Read the model definition and answer for the solid it produces. Units are mm, in the model's axes. Give positions to 0.01 mm unless a question says otherwise; leave off trailing zeros. Write each loop counter-clockwise with the first axis right and the second up, starting at its lowest first coordinate (ties: lowest second). Pieces come first, ordered by that corner, then holes. Notation, with made-up numbers: (75, 7.25) -> (121, 7.25) arc R27 cw to (121, 31.25) -> close; hole circle Ø9 at (75.5, 21.25). An arc over 180 degrees is marked (long way). Write item = value, one per line.
from build123d import *

# Parameters (mm, degrees)
F0_R     = 117.5
F0_R_2   = 11
F0_R_3   = 21.5
F1_DEPTH = 5
F2_R     = 7
F3_DEPTH = 5.001
F4_R     = 4
F5_DEPTH = 5.001


with BuildPart() as f1:
    # F0 (on Top) → F1 (new body)
    with BuildSketch(Plane.XY):
        Circle(F0_R)
        with Locations((7, -36)):
            Circle(F0_R_2, mode=Mode.SUBTRACT)
        with Locations((-17, 0)):
            Circle(F0_R_3, mode=Mode.SUBTRACT)
        with Locations((7, 36)):
            Circle(F0_R_2, mode=Mode.SUBTRACT)
    extrude(amount=F1_DEPTH)

    # F2 (on face) → F3 (cut, through all)
    with BuildSketch(Plane(origin=(0, 0, 0), x_dir=(1, 0, 0), z_dir=(0, 0, -1))):
        with Locations((-100, 0)):
            Circle(F2_R)
        with Locations((0, 100)):
            Circle(F2_R)
        with Locations((100, 0)):
            Circle(F2_R)
        with Locations((0, -100)):
            Circle(F2_R)
    extrude(amount=-F3_DEPTH, mode=Mode.SUBTRACT)

    # F4 (on face) → F5 (cut, through all)
    with BuildSketch(Plane.XY.offset(5)):
        with Locations((38, 0)):
            Circle(F4_R)
    extrude(amount=-F5_DEPTH, mode=Mode.SUBTRACT)


solid = f1.part
(1) The part is cut by section D-D on x = -43.5. Determine the outline of the cut face in (y, z).
Checks:
outline = (-109.15, 0) -> (109.15, 0) -> (109.15, 5) -> (-109.15, 5) -> close
(2) The part is cut by section A-A on x = -17. Determine the outline of the cut face in (y, z), plus the area to 3 significant figures.
Checks:
outline = (-116.26, 0) -> (-21.5, 0) -> (-21.5, 5) -> (-116.26, 5) -> close; (21.5, 0) -> (116.26, 0) -> (116.26, 5) -> (21.5, 5) -> close
area = 948 mm²
(3) For a pull along Y with two mould halves and no side action, classify faces 1 (the cylindrical face through (-0.91, 93.06, 2.46)), 2 (the flat face through (24, 2, 0)), 3 (the cylindrical face through (-15.3, 116.5, 2.5)) as released by +Y, released by -Y, zero draft, split by the parting line, or undercut.
Checks:
face_1 = undercut
face_2 = zero draft
face_3 = split by the parting line
(4) Consider L1, parallel to X at y = 6, z = 1.1; L2, parallel to Y at x = 9, z = 2.5; L3, parallel to X at y = -1.5, z = 3.5. Determine where each line is inside the solid, lowest interval first.
Checks:
L1 = -117.35 to -103.61, -96.39 to -37.65, 3.65 to 96.39, 103.61 to 117.35
L2 = -117.15 to -46.82, -25.18 to 25.18, 46.82 to 117.15
L3 = -117.49 to -106.84, -93.16 to -38.45, 4.45 to 34.29, 41.71 to 93.16, 106.84 to 117.49
(5) Given P1, Ø3, axis at y = 30.5, z = 4, coming from the -X side, flat-ended and moving along its own axis, determine where the tip first touches the part or whether it passes through.
Checks:
P1 = -113.87
(6) The part is cut by section B-B on y = -100. Determine the outline of the cut face in (x, z).
Checks:
outline = (-61.69, 0) -> (-7, 0) -> (-7, 5) -> (-61.69, 5) -> close; (7, 0) -> (61.69, 0) -> (61.69, 5) -> (7, 5) -> close
(7) The part is cut by section C-C on z = 3.3. Count the separate pieces of the cut face and the enclosed holes in it, plus the area to 3 significant figures.
Checks:
separate_pieces = 1
enclosed_holes = 8
area = 40,500 mm²
